Verification items for the finished model (mm, model axes). Face numbers are marked on the shaded views. A direction names the side the tool comes from. Coordinates: 2 decimals unless noted, no trailing zeros. Write each loop counter-clockwise with the first axis right and the second up, starting at its lowest first coordinate (ties: lowest second). Pieces come first, ordered by that corner, then holes. Notation, with made-up numbers: (59.5, 62) - (65.5, 62) arc R15 ccw to (65.5, 87) - close; hole circle Ø7 at (7.5, 19). An arc over 180 degrees is marked (long way). Use one line per item in the form item = value. Start each with the question number.
(1) Gauge pin test, flat ends, axial feed: pin 1 Ø6 at (y, z) = (28, -7) entering from -X; pin 2 Ø2 at (x, y) = (15.5, 2.5) entering from +Z; pin 3 Ø5 at (x, y) = (7, -3) entering from -Z. Record the tip position at first contact, or that the pin passes through.
(2) Sectioned sample at B-B (x = 3). Record the cut outline in (y, z).
(3) Sectioned sample at C-C (y = 2). Record the cut outline in (x, z).
(4) Sectioned sample at D-D (x = 13.75). Count the separate pieces of the cut face and the enclosed holes in it, and give its area (3 significant figures).
(5) Material ranges on line 1 (Z direction, x = 14, y = 1); line 2 (Y direction, x = 13, z = -7.75); line 3 (Z direction, x = 13.75, y = 21.5), recorded low to high. Write a range as [from, to].
(6) Mould release check, pull along Z, two halves, no side actions. Record for the marked faces 1, 2 and 3: released by +Z, released by -Z, zero draft, split by the parting line, or undercut.
(7) Sectioned sample at A-A (z = 6.5). Record the cut outline in (x, y), and give its area (3 significant figures).
(8) Tool access check on the marked faces 4, 5, 6 and 7. Record the directions out of +Z, -Z, +X, -X, +Y, -Y that give a thin tool (end or side, any length) a straight path to the whole face; none if there is none.
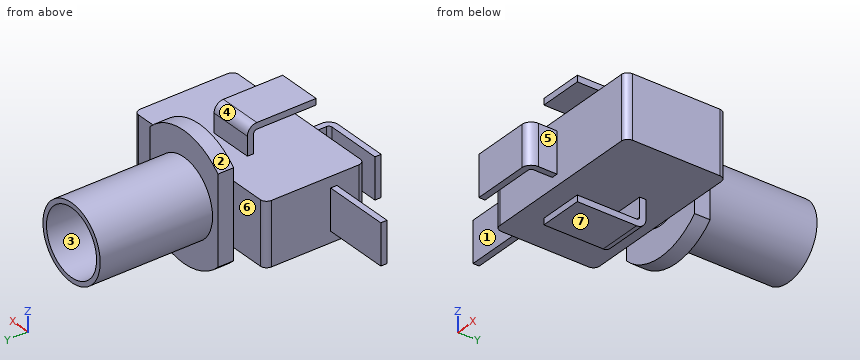
from build123d import *

# Parameters (mm, degrees)
BOSS_EXTRUDE1_DEPTH      = 5
BOSS_EXTRUDE1_DEPTH_BACK = 5
BOSS_EXTRUDE2_DEPTH      = 2.5
SKETCH3_W                = 1
SKETCH3_H                = 6.5
SKETCH6_W                = 6.5
SKETCH6_H                = 1
BOSS_EXTRUDE3_DEPTH      = 10.5
SKETCH7_W                = 7
SKETCH7_H                = 1
SKETCH9_R                = 6
BOSS_EXTRUDE4_DEPTH      = 18
SKETCH10_R               = 5.25
CUT_EXTRUDE1_DEPTH       = 20.5


with BuildPart() as part:
    # Sketch1 → Boss-Extrude1 (new body, two sides)
    with BuildSketch(Plane.XY) as boss_extrude1_sk:
        with BuildLine():
            Line((0, 1), (0, 15))
            ThreePointArc((0, 15), (0.292893219, 15.707106781), (1, 16))
            Line((1, 16), (26.5, 16))
            ThreePointArc((26.5, 16), (27.207106781, 15.707106781), (27.5, 15))
            Line((27.5, 15), (27.5, 1))
            ThreePointArc((27.5, 1), (27.207106781, 0.292893219), (26.5, 0))
            Line((26.5, 0), (1, 0))
            ThreePointArc((1, 0), (0.292893219, 0.292893219), (0, 1))
        make_face()
    extrude(amount=BOSS_EXTRUDE1_DEPTH)
    extrude(boss_extrude1_sk.sketch, amount=-BOSS_EXTRUDE1_DEPTH_BACK)

    # Sketch2 → Boss-Extrude2 (add)
    with BuildSketch(Plane(origin=(0, 16, 0), x_dir=(-1, 0, 0), z_dir=(0, 1, 0))):
        with BuildLine():
            Line((-20.891428429, 7), (-20.891428429, -7))
            ThreePointArc((-20.891428429, -7), (-13.75, -10), (-6.608571571, -7))
            Line((-6.608571571, -7), (-6.608571571, 7))
            ThreePointArc((-6.608571571, 7), (-13.75, 10), (-20.891428429, 7))
        make_face()
    extrude(amount=BOSS_EXTRUDE2_DEPTH)

    # Sweep1: sweep along a path in Sketch5
    with BuildLine(Plane.XY.offset(5)) as sweep1_path:
        Line((12, 0), (12, -3))
        ThreePointArc((12, -3), (11.853553391, -3.353553391), (11.5, -3.5))
        Line((11.5, -3.5), (2.5, -3.5))
    # Sketch3 → Sweep1 (sweep)
    with BuildSketch(Plane.XZ):
        with Locations((12.5, 0)):
            Rectangle(SKETCH3_W, SKETCH3_H)
    sweep(path=sweep1_path.line)

    # Sketch6 → Boss-Extrude3 (add)
    with BuildSketch(Plane.ZY):
        with Locations((0, 5)):
            Rectangle(SKETCH6_W, SKETCH6_H)
    extrude(amount=BOSS_EXTRUDE3_DEPTH)

    # Sweep2: sweep along a path in Sketch8
    with BuildLine(Plane.ZY) as sweep2_path:
        Line((5, 10), (8, 10))
        ThreePointArc((8, 10), (8.353553391, 9.853553391), (8.5, 9.5))
        Line((8.5, 9.5), (8.5, 0))
    # Sketch7 → Sweep2 (sweep)
    with BuildSketch(Plane.XY.offset(5)):
        with Locations((13.75, 10.5)):
            Rectangle(SKETCH7_W, SKETCH7_H)
    sweep2 = sweep(path=sweep2_path.line)

    # Mirror1: Sweep2 across plane
    add(sweep2.mirror(Plane.XY))

    # Sketch9 → Boss-Extrude4 (add)
    with BuildSketch(Plane(origin=(0, 18.5, 0), x_dir=(-1, 0, 0), z_dir=(0, 1, 0))):
        with Locations((-13.75, 0)):
            Circle(SKETCH9_R)
    extrude(amount=BOSS_EXTRUDE4_DEPTH)

    # Sketch10 → Cut-Extrude1 (cut)
    with BuildSketch(Plane(origin=(0, 36.5, 0), x_dir=(1, 0, 0), z_dir=(0, 1, 0))):
        with Locations((13.75, 0)):
            Circle(SKETCH10_R)
    extrude(amount=-CUT_EXTRUDE1_DEPTH, mode=Mode.SUBTRACT)


solid = part.part
Answers below:
q1.pin_1 = 9.28
q1.pin_2 = 9.5
q1.pin_3 = -3.25
q2.outline = (-4.5, -3.25) - (-3.5, -3.25) - (-3.5, 3.25) - (-4.5, 3.25) - close; (0, -5) - (16, -5) - (16, 5) - (0, 5) - close
q3.outline = (0, -5) - (27.5, -5) - (27.5, 5) - (0, 5) - close; (10.25, -9.5) - (17.25, -9.5) - (17.25, -8.5) - (10.25, -8.5) - close; (10.25, 8.5) - (17.25, 8.5) - (17.25, 9.5) - (10.25, 9.5) - close
q4.separate_pieces = 3
q4.enclosed_holes = 0
q4.area = 239 mm2
q5.line_1 = [-9.5, -8.5], [-5, 5], [8.5, 9.5]
q5.line_2 = [10, 11], [16, 18.5]
q5.line_3 = [-6, -5.25], [5.25, 6]
q6.face_1 = zero draft
q6.face_2 = released by +Z
q6.face_3 = undercut
q7.outline = (6.61, 16) - (20.89, 16) - (20.89, 18.5) - (6.61, 18.5) - close; (10.25, 10) - (17.25, 10) - (17.25, 11) - (10.25, 11) - close
q7.area = 42.7 mm2
q8.face_4 = +Z, +X, -X
q8.face_5 = +Z, -Z, +X, -Y
q8.face_6 = +Z, -Z, -X, +Y
q8.face_7 = -Z, +X, -X, -Y
